```python
from build123d import *

# Parameters (mm, degrees)
SKETCH_1_W          = 170
SKETCH_1_H          = 180
EXTRUDE_1_DEPTH     = 10
SKETCH_2_R          = 50
SKETCH_2_R_2        = 2.75
SKETCH_2_R_3        = 2.1
SKETCH_2_R_4        = 3.25
CUT_EXTRUDE_1_DEPTH = 11


with BuildPart() as part:
    # 草图1 → 凸台-拉伸1 (new body)
    with BuildSketch(Plane.XY):
        with Locations((5, 0)):
            Rectangle(SKETCH_1_W, SKETCH_1_H)
    extrude(amount=EXTRUDE_1_DEPTH)

    # 草图2 → 切除-拉伸1 (cut)
    with BuildSketch(Plane(origin=(0, 0, 0), x_dir=(-1, 0, 0), z_dir=(0, 0, -1))):
        Circle(SKETCH_2_R)
        with Locations((-56, 0)):
            Circle(SKETCH_2_R_2)
        with Locations((-48.497422612, 28)):
            Circle(SKETCH_2_R_2)
        with Locations((-28, 48.497422612)):
            Circle(SKETCH_2_R_2)
        with Locations((0, 56)):
            Circle(SKETCH_2_R_2)
        with Locations((28, 48.497422612)):
            Circle(SKETCH_2_R_2)
        with Locations((48.497422612, 28)):
            Circle(SKETCH_2_R_2)
        with Locations((56, 0)):
            Circle(SKETCH_2_R_2)
        with Locations((48.497422612, -28)):
            Circle(SKETCH_2_R_2)
        with Locations((28, -48.497422612)):
            Circle(SKETCH_2_R_2)
        with Locations((0, -56)):
            Circle(SKETCH_2_R_2)
        with Locations((-28, -48.497422612)):
            Circle(SKETCH_2_R_2)
        with Locations((-48.497422612, -28)):
            Circle(SKETCH_2_R_2)
        with Locations((-52.622786764, 19.153128026)):
            Circle(SKETCH_2_R_3)
        with Locations((19.153128026, 52.622786764)):
            Circle(SKETCH_2_R_3)
        with Locations((52.622786764, -19.153128026)):
            Circle(SKETCH_2_R_3)
        with Locations((-19.153128026, -52.622786764)):
            Circle(SKETCH_2_R_3)
        with Locations((-62, -80)):
            Circle(SKETCH_2_R_4)
        with Locations((-62, -50)):
            Circle(SKETCH_2_R_4)
        with Locations((-62, 50)):
            Circle(SKETCH_2_R_4)
        with Locations((-62, 80)):
            Circle(SKETCH_2_R_4)
    extrude(amount=-CUT_EXTRUDE_1_DEPTH, mode=Mode.SUBTRACT)


solid = part.part
```
Work out the finished part from the listing and answer in its coordinate system (mm). Round coordinates to 2 decimals unless told otherwise and drop trailing zeros. Loops run counter-clockwise (first coordinate to the right, second up) from the corner with the lowest first, then second, coordinate; pieces in that order, holes last.
(1) This flat-tipped pin is pushed along its axis until it touches: P1, Ø4.5, axis at x = 48.5, y = -28, coming from the -Z side. Where does it stop, or does it pass through?
Computed values:
P1: passes through
(2) Find the intervals of material crossed by L1, parallel to X at y = -51, z = 7.5; L2, parallel to Y at x = 62, z = 5.75; L3, parallel to Y at x = 17.5, z = 9, in increasing order.
Computed values:
L1: x = -80 to -29.14, -26.86 to 17.82, 20.49 to 26.86, 29.14 to 58.91, 65.09 to 90
L2: y = -90 to -83.25, -76.75 to -53.25, -46.75 to 46.75, 53.25 to 76.75, 83.25 to 90
L3: y = -90 to -53.92, -51.33 to -46.84, 46.84 to 90
(3) The mould has two halves that part along X. Classify faces 1 (the flat face through (-34, 41, 0)), 2 (the cylindrical face through (64.579, -81.978, 4.93)), 3 (the flat face through (-80, -1, 5)): pulls with the +X half, pulls with the -X half, needs draft (parallel to the pull), parting line crosses it, or undercut.
Computed values:
face 1: needs draft
face 2: undercut
face 3: pulls with the -X half
(4) The part is cut by section D-D, the plane z = 5.25. Give the number of separate pieces and of enclosed holes in the cut face, and give its area (3 significant figures).
Computed values:
separate pieces: 1
enclosed holes: 21
area: 22,300 mm2
(5) The part is cut by section C-C, the plane y = 0. Give the vertices of the cut face in (x, z).
Computed values:
outline: (-80, 0) - (-58.75, 0) - (-58.75, 10) - (-80, 10) - close; (-53.25, 0) - (-50, 0) - (-50, 10) - (-53.25, 10) - close; (50, 0) - (53.25, 0) - (53.25, 10) - (50, 10) - close; (58.75, 0) - (90, 0) - (90, 10) - (58.75, 10) - close
(6) The part is cut by section A-A, the plane y = -80. Give the vertices of the cut face in (x, z).
Computed values:
outline: (-80, 0) - (58.75, 0) - (58.75, 10) - (-80, 10) - close; (65.25, 0) - (90, 0) - (90, 10) - (65.25, 10) - close
(7) The part is cut by section B-B, the plane x = -28. Give the vertices of the cut face in (y, z).
Computed values:
outline: (-90, 0) - (-51.25, 0) - (-51.25, 10) - (-90, 10) - close; (-45.75, 0) - (-41.42, 0) - (-41.42, 10) - (-45.75, 10) - close; (41.42, 0) - (45.75, 0) - (45.75, 10) - (41.42, 10) - close; (51.25, 0) - (90, 0) - (90, 10) - (51.25, 10) - close
